from build123d import *

# Parameters (mm, degrees)
SKETCH1_W           = 42
SKETCH1_H           = 20
SKETCH1_R           = 6.75
BOSS_EXTRUDE1_DEPTH = 5
SKETCH1_3_R         = 6.75
BOSS_EXTRUDE2_DEPTH = 85
SKETCH2_R           = 9.5
BOSS_EXTRUDE3_DEPTH = 6
FILLET1_R           = 1


with BuildPart() as part:
    # Sketch1 → Boss-Extrude1 (new body)
    # profile 1 of 3: a face of its own
    with BuildSketch(Plane(origin=(0, 0, 0), x_dir=(1, 0, 0), z_dir=(0, 1, 0))):
        Rectangle(SKETCH1_W, SKETCH1_H)
        with Locations((10.5, 0)):
            Circle(SKETCH1_R, mode=Mode.SUBTRACT)
        with Locations((-10.5, 0)):
            Circle(SKETCH1_R, mode=Mode.SUBTRACT)
    # profile 2 of 3: a face of its own
    with BuildSketch(Plane(origin=(0, 0, 0), x_dir=(1, 0, 0), z_dir=(0, 1, 0))):
        with Locations((10.5, 0)):
            Circle(SKETCH1_R)
    # profile 3 of 3: a face of its own
    with BuildSketch(Plane(origin=(0, 0, 0), x_dir=(1, 0, 0), z_dir=(0, 1, 0))):
        with Locations((-10.5, 0)):
            Circle(SKETCH1_R)
    extrude(amount=BOSS_EXTRUDE1_DEPTH)

    # Sketch1_3 → Boss-Extrude2 (add)
    with BuildSketch(Plane(origin=(0, 0, 0), x_dir=(1, 0, 0), z_dir=(0, 1, 0))):
        with Locations(Location((-10.5, 0, 0), (0, 0, 270))):
            Circle(SKETCH1_3_R)
        with Locations(Location((10.5, 0, 0), (0, 0, 270))):
            Circle(SKETCH1_3_R)
    extrude(amount=BOSS_EXTRUDE2_DEPTH)

    # Sketch2 → Boss-Extrude3 (add)
    with BuildSketch(Plane(origin=(0, 85, 0), x_dir=(1, 0, 0), z_dir=(0, 1, 0))):
        with Locations(Location((-10.5, 0, 0), (0, 0, 270))):
            Circle(SKETCH2_R)
    extrude(amount=-BOSS_EXTRUDE3_DEPTH)

    # Fillet1
    fillet1_edges = [part.edges().sort_by_distance(p)[0] for p in [
        (0, 5, -10),
        (-21, 5, 0),
        (0, 5, 10),
        (-10.5, 79, -6.75),
        (-10.5, 79, -9.5),
        (21, 5, 0),
        (0, 0, 10),
        (-21, 0, 0),
        (0, 0, -10),
        (21, 2.5, 10),
        (-21, 2.5, 10),
        (-21, 2.5, -10),
        (21, 2.5, -10),
    ]]
    fillet(fillet1_edges, radius=FILLET1_R)


solid = part.part
Part model, mm, in its own coordinate system. A direction names the side the tool comes from. Coordinates: 2 decimals unless noted, no trailing zeros. Loops run counter-clockwise (first coordinate to the right, second up) from the corner with the lowest first, then second, coordinate; pieces in that order, holes last. Notation, with made-up numbers: M -20,70 L -6,70 A19 cw -6,88 Z; hole C 72.25,11 d9. An arc over 180 degrees is marked long. Use a Markdown table: item, result. Add a question column.
Q1. Cut at A-A (x = -10.5). Write the cut outline in (y, z).
Q2. Cut at C-C (y = 62). Write the cut outline in (x, z), and give its area (3 significant figures).
Q3. Probe L1, parallel to Z at x = -11, y = 59; L2, parallel to Y at x = 2, z = 8; L3, parallel to Y at x = -14, z = -6.5. List the from-to ranges inside material, lowest first.
Q4. Cut at B-B (z = 0). Write the cut outline in (x, y), and give its area (3 significant figures).
Q5. Pin check, flat tips, straight feed: P1, Ø1, axis at x = -6, y = 64.5, coming from the -Z side; P2, Ø1.5, axis at y = 54, z = 7, coming from the -X side; P3, Ø1.5, axis at y = 12, z = -5.5, coming from the +X side. Stop position of each tip, or through.
Q6. Which spindle directions (+Z, -Z, +X, -X, +Y, -Y) get a long thin tool onto all of the face, cutting with end or side? Do faces 1 (the flat face through (0, 5, 0)), 2 (the flat face through (1, 0, 0)), 3 (the cylindrical face through (16.19, 44.44, 3.63)). Say none if no direction does.
Q7. Cut at D-D (x = 10.5). Write the cut outline in (y, z), and give its area (3 significant figures).
Q8. Mould opens along X. For faces 4 (the flat face through (11, 85, 0)), 5 (the cylindrical face through (-16.49, 40.99, 3.11)), 6 (the flat face through (-21, 2, 0)) say: +X half, -X half, draft (parallel to the pull), parting line (faces both ways), or undercut.
Worked out:
| question | item | result |
|---|---|---|
| 1 | outline | M 0,-9 A1 ccw 1,-10 L 4,-10 A1 ccw 5,-9 L 5,-6.75 L 78,-6.75 A1 cw 79,-7.75 L 79,-8.5 A1 ccw 80,-9.5 L 85,-9.5 L 85,9.5 L 80,9.5 A1 ccw 79,8.5 L 79,7.75 A1 cw 78,6.75 L 5,6.75 L 5,9 A1 ccw 4,10 L 1,10 A1 ccw 0,9 Z |
| 2 | outline | C -10.5,0 d13.5; C 10.5,0 d13.5 |
| 2 | area | 286 mm2 |
| 3 | L1 | z = -6.73 to 6.73 |
| 3 | L2 | y = 0 to 5 |
| 3 | L3 | y = 0 to 5, 78.93 to 85 |
| 4 | outline | M -21,1 A1 ccw -20,0 L 21,0 L 21,4 A1 ccw 20,5 L 17.25,5 L 17.25,85 L 3.75,85 L 3.75,5 L -3.75,5 L -3.75,78 A1 cw -2.75,79 L -2,79 A1 ccw -1,80 L -1,85 L -20,85 L -20,80 A1 ccw -19,79 L -18.25,79 A1 cw -17.25,78 L -17.25,5 L -20,5 A1 ccw -21,4 Z |
| 4 | area | 2,400 mm2 |
| 5 | P1 | stops at z = -5.44 |
| 5 | P2 | stops at x = -13.05 |
| 5 | P3 | stops at x = 15.3 |
| 6 | face 1 | none |
| 6 | face 2 | +Z, -Z, +X, -X, -Y |
| 6 | face 3 | +Y |
| 7 | outline | M 0,-9 A1 ccw 1,-10 L 4,-10 A1 ccw 5,-9 L 5,-6.75 L 85,-6.75 L 85,6.75 L 5,6.75 L 5,9 A1 ccw 4,10 L 1,10 A1 ccw 0,9 Z |
| 7 | area | 1,180 mm2 |
| 8 | face 4 | draft |
| 8 | face 5 | undercut |
| 8 | face 6 | -X half |
